Could you check a few things on this model? Use its own coordinates, in mm. Round coordinates to 2 decimals unless told otherwise and drop trailing zeros. Loops run counter-clockwise (first coordinate to the right, second up) from the corner with the lowest first, then second, coordinate; pieces in that order, holes last. Notation, with made-up numbers: (83, -24.5) - (127, -24.5) arc R27 ccw to (127, -7.5) - close; hole circle Ø7 at (-27.5, -4.5). An arc over 180 degrees is marked (long way). Use one line per item in the form item = value.
```python
from build123d import *

# Parameters (mm, degrees)
SKETCH_1_R               = 3
EXTRUDE_1_DEPTH          = 60
CHAMFER_1_SIZE           = 2
SKETCH_2_R               = 0.75
CUT_EXTRUDE_1_DEPTH      = 4
CUT_EXTRUDE_1_DEPTH_BACK = 4


with BuildPart() as part:
    # Эскиз1 → Бобышка-Вытянуть1 (new body)
    with BuildSketch(Plane(origin=(0, 0, 0), x_dir=(0, 0, -1), z_dir=(1, 0, 0))):
        Circle(SKETCH_1_R)
    extrude(amount=EXTRUDE_1_DEPTH)

    # Фаска1
    chamfer_1_edges = [part.edges().sort_by_distance(p)[0] for p in [
        (0, 0, 3),
        (60, 0, 3),
    ]]
    chamfer(chamfer_1_edges, length=CHAMFER_1_SIZE)

    # Эскиз2 → Вырез-Вытянуть1 (cut, two sides)
    with BuildSketch(Plane.XY) as cut_extrude_1_sk:
        with Locations((5, 0)):
            Circle(SKETCH_2_R)
        with Locations((55, 0)):
            Circle(SKETCH_2_R)
    extrude(amount=CUT_EXTRUDE_1_DEPTH, mode=Mode.SUBTRACT)
    extrude(cut_extrude_1_sk.sketch, amount=-CUT_EXTRUDE_1_DEPTH_BACK, mode=Mode.SUBTRACT)


solid = part.part
```
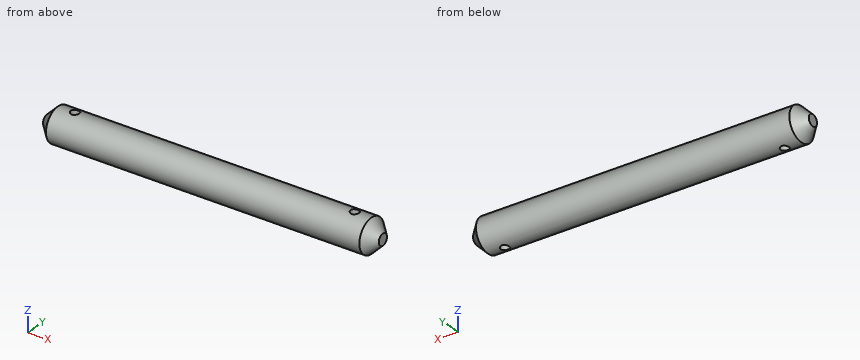
1. If we section it at B-B, the plane y = 0: Write out the boundary of the cut face in (x, z), plus the area to 3 significant figures.
Solution:
outline = (0, -1) - (2, -3) - (4.25, -3) - (4.25, 3) - (2, 3) - (0, 1) - close; (5.75, -3) - (54.25, -3) - (54.25, 3) - (5.75, 3) - close; (55.75, -3) - (58, -3) - (60, -1) - (60, 1) - (58, 3) - (55.75, 3) - close
area = 334 mm^2
2. For P1, Ø1.5, axis at x = 52.5, y = 1.5, coming from the +Z side; P2, Ø3, axis at y = -2.5, z = -1, coming from the +X side, each with a flat end and sliding along its axis, tell me the tip position at first contact or that it passes through.
Solution:
P1 = 2.9
P2 = 59.81
3. If we section it at C-C, the plane x = 5: Write out the boundary of the cut face in (y, z).
Solution:
outline = (-0.75, -2.9) - (-0.75, 2.9) arc R3 ccw to start; (0.75, -2.9) arc R3 ccw to (0.75, 2.9) - close
4. Please list where these lines run through material, in increasing order: line 1 along X through (y, z) = (0, 0.75); line 2 along X through (y, z) = (0, 1.5); line 3 along Y through (x, z) = (55, -0.25).
Solution:
line_1 = 0 to 4.25, 5.75 to 54.25, 55.75 to 60
line_2 = 0.5 to 4.25, 5.75 to 54.25, 55.75 to 59.5
line_3 = -2.99 to -0.75, 0.75 to 2.99
5. If we section it at A-A, the plane z = 0: Write out the boundary of the cut face in (x, y).
Solution:
outline = (0, -1) - (2, -3) - (58, -3) - (60, -1) - (60, 1) - (58, 3) - (2, 3) - (0, 1) - close; hole circle Ø1.5 at (5, 0); hole circle Ø1.5 at (55, 0)
6. If we section it at D-D, the plane x = 22.5: Write out the boundary of the cut face in (y, z).
Solution:
outline = circle Ø6 at (0, 0)
